Answer from the drawing. Dimensions are ordinates in mm from the lowest x, y and z of the part. A direction names the side the tool comes from. Round coordinates to 2 decimals unless told otherwise and drop trailing zeros. Order: outer loops, then holes, each group sorted by start corner. A loop starts at its lowest first (then second) coordinate and runs counter-clockwise, first axis right, second up. Notation, with made-up numbers: (44, 35) -> (58, 35) arc R18 cw to (58, 65) -> close; hole circle Ø5 at (9, 8.25). An arc over 180 degrees is marked (long way). Use a Markdown table: item, result. Add a question column.
Item 1: A cutting plane is placed at A-A, the plane x = 3. Determine the outline of the cut face in (y, z), plus the area to 3 significant figures.
Item 2: A tool of negligible diameter and unlimited length cuts with its end or side. For the marked faces 4 and 5, from which of +Z, -Z, +X, -X, +Y, -Y can it reach the whole face along a straight path? Write none if from no direction.
Item 3: Flat-ended cylindrical pins translate along their axes: P1, Ø0.6, axis at x = 3, z = 0.5, coming from the +Y side; P2, Ø0.6, axis at x = 3, z = 0.5, coming from the -Y side; P3, Ø1, axis at x = 2.5, z = 4.5, coming from the +Y side. Find the tip coordinate at first contact, or state that the pin passes through.
Item 4: A cutting plane is placed at B-B, the plane z = 3. Determine the outline of the cut face in (x, y).
Item 5: Find the intervals of material crossed by L1, parallel to Z at x = 2.5, y = 3.5; L2, parallel to X at y = 3.15, z = 6; L3, parallel to Z at x = 0.6, y = 3.45, in increasing order. Write a range as [from, to].
Item 6: For a pull along X with two mould halves and no side action, classify the marked faces 1, 2 and 3 as +X half, -X half, draft (parallel to the pull), parting line (faces both ways), or undercut.
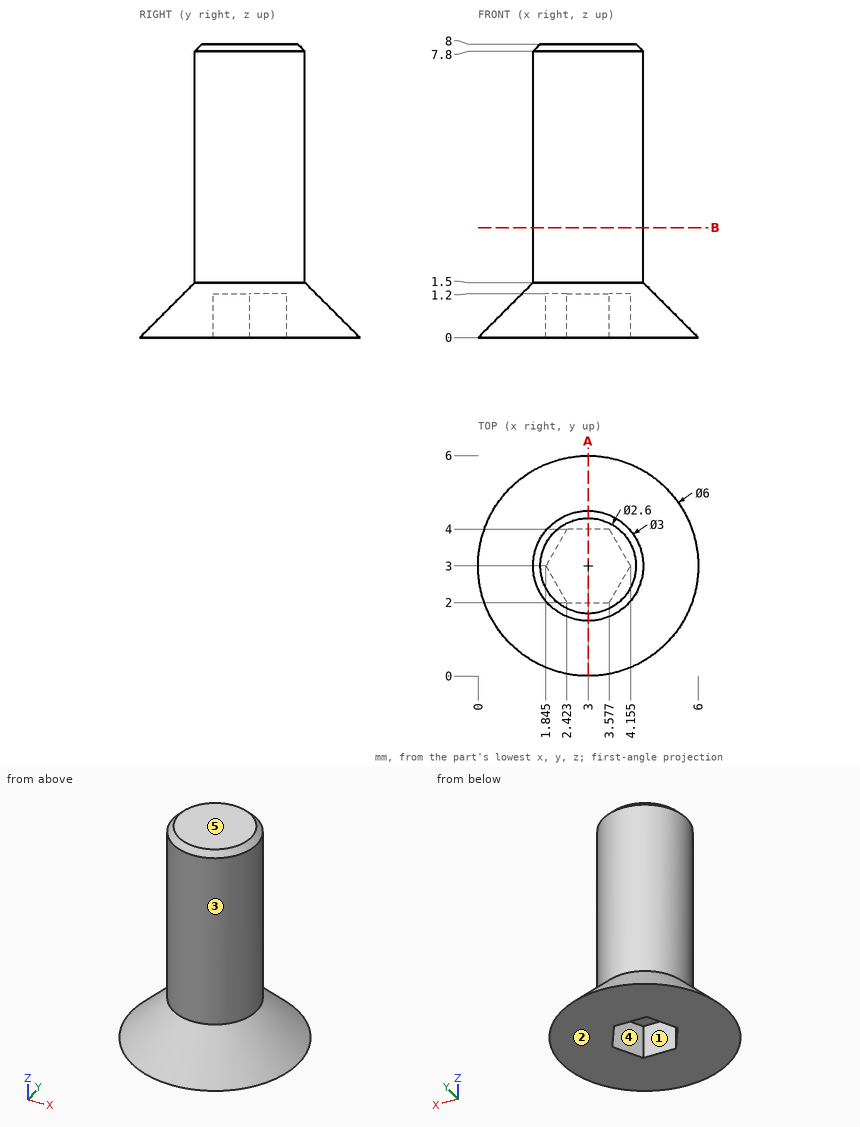
Reported:
| question | item | result |
|---|---|---|
| 1 | outline | (0, 0) -> (2, 0) -> (2, 1.2) -> (4, 1.2) -> (4, 0) -> (6, 0) -> (4.5, 1.5) -> (4.5, 7.8) -> (4.3, 8) -> (1.7, 8) -> (1.5, 7.8) -> (1.5, 1.5) -> close |
| 1 | area | 23.8 mm² |
| 2 | face 4 | -Z |
| 2 | face 5 | +Z, +X, -X, +Y, -Y |
| 3 | P1 | y = 5.8 |
| 3 | P2 | y = 0.2 |
| 3 | P3 | y = 4.5 |
| 4 | outline | circle Ø3 at (3, 3) |
| 5 | L1 | [1.2, 8] |
| 5 | L2 | [1.51, 4.49] |
| 5 | L3 | [0, 0.56] |
| 6 | face 1 | undercut |
| 6 | face 2 | draft |
| 6 | face 3 | parting line |
